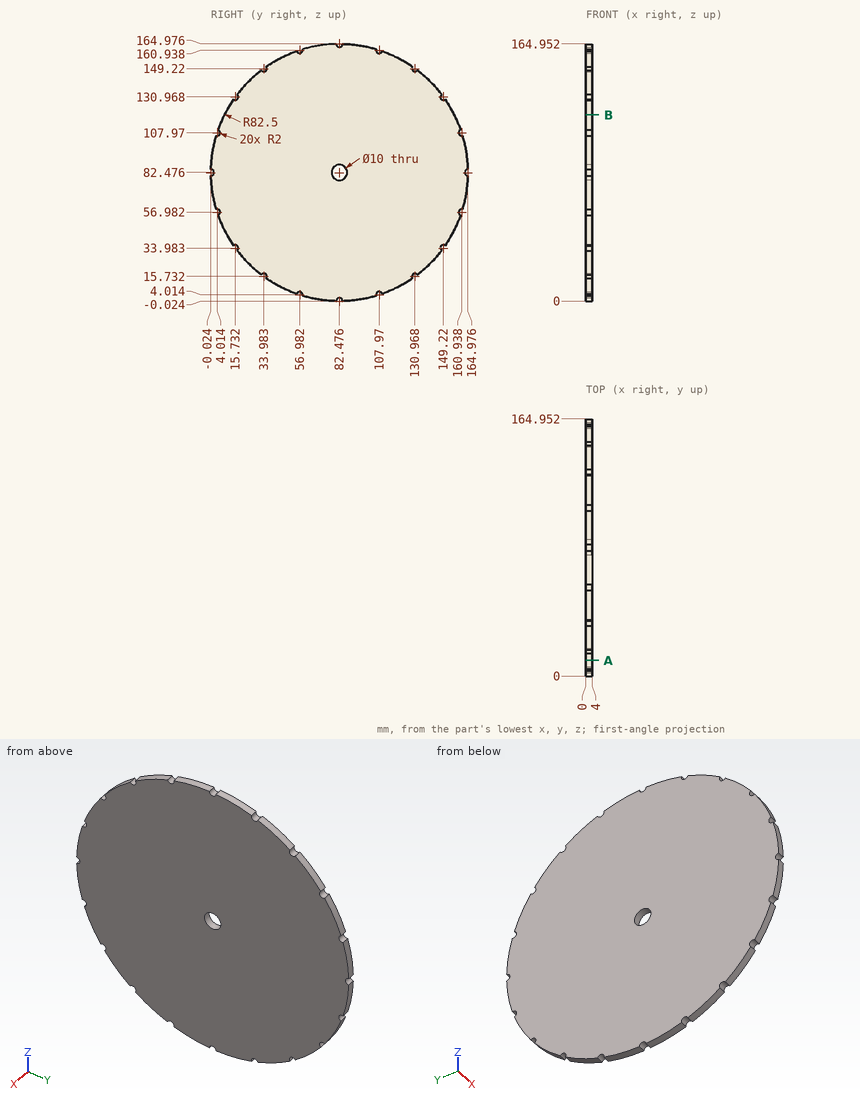
Verification items for this drawing (mm, ordinates from the low corner). Coordinates: 2 decimals unless noted, no trailing zeros. Write each loop counter-clockwise with the first axis right and the second up, starting at its lowest first coordinate (ties: lowest second). Pieces come first, ordered by that corner, then holes. Notation, with made-up numbers: M 45,87.5 L 96,87.5 A26 cw 96,119.5 Z; hole C 19,-38.75 d5. An arc over 180 degrees is marked long. Use CSV: the item, a comma, the result in double quotes.
Q1. Go/stop test with flat-tipped pins: P1, Ø2, axis at x = 0.5, y = 97, coming from the -Z side; P2, Ø2, axis at x = 1.5, y = 100.5, coming from the -Z side. Record where each tip stops, or that it passes through.
Computed values:
P1,"z = 1.09"
P2,"z = 1.75"
Q2. Section check A-A, the plane y = 10. Enter the section's corners in (x, z).
Computed values:
outline,"M 0,43.06 L 4,43.06 L 4,121.89 L 0,121.89 Z"
Q3. Thickness scan on line 1 along Z through (x, y) = (0.8, 83) (1 decimal); line 2 along Z through (x, y) = (2.75, 65.5); line 3 along Y through (x, z) = (1.6, 22.5) (1 decimal). Record the ranges inside material, lowest first. Write a range as [from, to].
Computed values:
line 1,"[1.9, 77.5], [87.4, 163]"
line 2,"[1.74, 163.21]"
line 3,"[25.8, 139.1]"
Q4. Section check B-B, the plane z = 119.5. Enter the section's corners in (x, y), and give its area (3 significant figures).
Computed values:
outline,"M 0,8.75 L 4,8.75 L 4,156.2 L 0,156.2 Z"
area,"590 mm²"
